```python
from build123d import *

# Parameters (mm, degrees)
F0_R     = 1.8
F0_W     = 25
F0_H     = 4.5
F0_R_2   = 1
F1_DEPTH = 2
F2_R     = 3
F3_DEPTH = 12
F4_R     = 0.5


with BuildPart() as f1:
    # F0 (on Top) → F1 (new body)
    with BuildSketch(Plane.XY):
        Polygon((-12.5, 17.5), (-19, 17.5), (-19, -17.5), (-12.5, -17.5), (-12.5, -13), (-12.5, 13), align=None)
        with Locations((-16, -14)):
            Circle(F0_R, mode=Mode.SUBTRACT)
        with Locations((-16, 14)):
            Circle(F0_R, mode=Mode.SUBTRACT)
        Polygon((19, 17.5), (12.5, 17.5), (12.5, 13), (12.5, -13), (12.5, -17.5), (19, -17.5), align=None)
        with Locations((16, -14)):
            Circle(F0_R, mode=Mode.SUBTRACT)
        with Locations((16, 14)):
            Circle(F0_R, mode=Mode.SUBTRACT)
        with Locations((0, 15.25)):
            Rectangle(F0_W, F0_H)
        with Locations((-6.5, 15.25)):
            Circle(F0_R_2, mode=Mode.SUBTRACT)
        with Locations((6.5, 15.25)):
            Circle(F0_R_2, mode=Mode.SUBTRACT)
        with Locations((0, -15.25)):
            Rectangle(F0_W, F0_H)
        with Locations((-8.25, -15.25)):
            Circle(F0_R_2, mode=Mode.SUBTRACT)
        with Locations((8.25, -15.25)):
            Circle(F0_R_2, mode=Mode.SUBTRACT)
    extrude(amount=F1_DEPTH)

    # F2
    f2_edges = [f1.edges().sort_by_distance(p)[0] for p in [
        (-19, 17.5, 1),
        (19, 17.5, 1),
        (19, -17.5, 1),
        (-19, -17.5, 1),
    ]]
    fillet(f2_edges, radius=F2_R)

    # F0 (on Top) → F3 (join)
    with BuildSketch(Plane.XY):
        with Locations((0, 15.25)):
            Rectangle(F0_W, F0_H)
        with Locations((-6.5, 15.25)):
            Circle(F0_R_2, mode=Mode.SUBTRACT)
        with Locations((6.5, 15.25)):
            Circle(F0_R_2, mode=Mode.SUBTRACT)
        with Locations((0, -15.25)):
            Rectangle(F0_W, F0_H)
        with Locations((-8.25, -15.25)):
            Circle(F0_R_2, mode=Mode.SUBTRACT)
        with Locations((8.25, -15.25)):
            Circle(F0_R_2, mode=Mode.SUBTRACT)
    extrude(amount=F3_DEPTH)

    # F4
    f4_edges = [f1.edges().sort_by_distance(p)[0] for p in [
        (-12.5, 15.25, 2),
        (-12.5, -15.25, 2),
        (12.5, 15.25, 2),
        (12.5, -15.25, 2),
    ]]
    fillet(f4_edges, radius=F4_R)


solid = f1.part
```
Model file for the job. Use its own axes, mm. A direction names the side the tool comes from. Coordinates: 2 decimals unless noted, no trailing zeros. Order: outer loops, then holes, each group sorted by start corner. A loop starts at its lowest first (then second) coordinate and runs counter-clockwise, first axis right, second up. Notation, with made-up numbers: (22, 24.25) - (71, 24.25) arc R5 cw to (71, 29.25) - close; hole circle Ø10 at (-20.75, -9). An arc over 180 degrees is marked (long way). Return JSON: item names as keys, results as strings. Group by question number.
1) Saw through at C-C, the plane x = 10. Write the cut outline in (y, z).
2) Tool access for faces 5 (the flat face through (0, -17.5, 6)), 6 (the flat face through (12.5, 0, 1)), 7 (the flat face through (12.5, -15, 7)), 8 (the flat face through (-12.5, 15, 7)): list every direction of +Z, -Z, +X, -X, +Y, -Y with a clear straight run to the whole face (end or side of a thin tool).
3) Saw through at D-D, the plane y = 2. Write the cut outline in (x, z).
4) Flat gauge pins, fed straight in: P1, Ø2, axis at y = -14.5, z = 6.5, coming from the -X side; P2, Ø6, axis at x = 16, y = 14, coming from the -Z side; P3, Ø12, axis at x = 10.5, y = -3, coming from the +Z side; P4, Ø5, axis at y = -15.5, z = 6, coming from the +X side. Where does each tip first touch, or does it go through?
5) Mould opens along Y. For faces 1 (the cylindrical face through (18.1, -16.64, 1.01)), 2 (the cylindrical face through (-6.717, 14.274, 5.916)), 3 (the flat face through (0, 13, 6)), 4 (the flat face through (-19, 0, 1)) say: released by +Y, released by -Y, zero draft, split by the parting line, or undercut.
6) Probe line 1 (Y direction, x = -6.5, z = 5.25); line 2 (Y direction, x = 16, z = 1.05); line 3 (Y direction, x = 11, z = 1). List the from-to ranges inside material, lowest first. Write a range as from..to.
7) Saw through at B-B, the plane y = -15.25. Write the cut outline in (x, z), plus the area to 3 significant figures.
8) Saw through at A-A, the plane z = 3.25. Write the cut outline in (x, y), plus the area to 3 significant figures.
Values found:
{
 "1": {"outline": "(-17.5, 0) - (-13, 0) - (-13, 12) - (-17.5, 12) - close; (13, 0) - (17.5, 0) - (17.5, 12) - (13, 12) - close"},
 "2": {"face 5": "+Z, -Z, +X, -X, -Y", "face 6": "+Z, -Z", "face 7": "+Z, +X, +Y, -Y", "face 8": "+Z, -X, +Y, -Y"},
 "3": {"outline": "(-19, 0) - (-12.5, 0) - (-12.5, 2) - (-19, 2) - close; (12.5, 0) - (19, 0) - (19, 2) - (12.5, 2) - close"},
 "4": {"P1": "stops at x = -12.5", "P2": "stops at z = 0", "P3": "stops at z = 2", "P4": "stops at x = 12.5"},
 "5": {"face 1": "released by -Y", "face 2": "undercut", "face 3": "undercut", "face 4": "zero draft"},
 "6": {"line 1": "y = -17.5..-13, 13..14.25, 16.25..17.5", "line 2": "y = -17.5..-15.8, -12.2..12.2, 15.8..17.5", "line 3": "y = -17.5..-13, 13..17.5"},
 "7": {"outline": "(-18.9, 0) - (-17.3, 0) - (-17.3, 2) - (-18.9, 2) - close; (-14.7, 0) - (-9.25, 0) - (-9.25, 12) - (-12.5, 12) - (-12.5, 2.5) arc R0.5 cw to (-13, 2) - (-14.7, 2) - close; (-7.25, 0) - (7.25, 0) - (7.25, 12) - (-7.25, 12) - close; (9.25, 0) - (14.7, 0) - (14.7, 2) - (13, 2) arc R0.5 cw to (12.5, 2.5) - (12.5, 12) - (9.25, 12) - close; (17.3, 0) - (18.9, 0) - (18.9, 2) - (17.3, 2) - close", "area": "267 mm²"},
 "8": {"outline": "(-12.5, -17.5) - (12.5, -17.5) - (12.5, -13) - (-12.5, -13) - close; (-12.5, 13) - (12.5, 13) - (12.5, 17.5) - (-12.5, 17.5) - close; hole circle Ø2 at (-8.25, -15.25); hole circle Ø2 at (-6.5, 15.25); hole circle Ø2 at (6.5, 15.25); hole circle Ø2 at (8.25, -15.25)", "area": "212 mm²"}
}
